Autodesk Inventor part; units mm, degrees
ref_plane "Work Plane1" through (0, 65, -37.4166) normal (0, 0, 1) x (1, 0, 0)
ref_plane "Work Plane2" through (0, 0, -75) normal (0, 0, 1) x (1, 0, 0)
ref_plane "Work Plane3" through (65, 0, -37.4166) normal (1, 0, 0) x (0, 1, 0)
sketch "Sketch1" plane through (0, 0, 0) normal (0, 0, 1) x (1, 0, 0)
  line L0 (65, -65) -> (-65, -65)
  line L1 (-65, -65) -> (-65, 65)
  line L2 (-65, 65) -> (65, 65)
  line L3 (65, 65) -> (65, -65)
  line L4 (65, -65) -> (-65, 65) construction
  line L5 (-65, -65) -> (65, 65) construction
  point P0 (0, 0)
  dimension "d0" = 130
  dimension "d1" = 130
extrude "Extrusion1" add sketch "Sketch1" against normal blind 100
sketch "Sketch2" plane through (0, 0, 0) normal (0, 0, 1) x (1, 0, 0)
  arc A0 (0, 75) -> (0, -75) centre (0, 0) ccw
  line L0 (0, 0) -> (0, 75) construction
  line L1 (0, 0) -> (75, 0) construction
  line L2 (0, 0) -> (0, -75) construction
  line L3 (0, 75) -> (0, -75)
  dimension "d4" = 75
  dimension "d5" = 90
  dimension "d6" = 180
revolve "Revolution1" cut sketch "Sketch2" angle 180 about axis through (0, 75, 0) along (0, -1, 0)
ref_plane "Work Plane1" through (0, 65, -37.4166) normal (0, 0, 1) x (1, 0, 0)
sketch "Sketch3" plane through (0, 65, -37.4166) normal (0, 0, 1) x (1, 0, 0)
  line L0 (-65, -130) -> (65, -130)
  line L1 (65, -130) -> (65, 0)
  line L2 (65, 0) -> (-65, 0)
  line L3 (-65, 0) -> (-65, -130)
  line L4 (-65, -130) -> (65, 0) construction
  line L5 (65, -130) -> (-65, 0) construction
  point P0 (0, -65)
  dimension "d8" = 130
  dimension "d9" = 130
extrude "Extrusion2" cut sketch "Sketch3" along normal blind 100
sketch "Sketch4" plane through (0, 65, -37.4166) normal (0, 0, 1) x (1, 0, 0)
  line L0 (-65, -130) -> (65, -130)
  line L1 (65, -130) -> (65, 0)
  line L2 (65, 0) -> (-65, 0)
  line L3 (-65, 0) -> (-65, -130)
  line L4 (-65, -130) -> (65, 0) construction
  line L5 (65, -130) -> (-65, 0) construction
  line L6 (-70, -135) -> (70, -135)
  line L7 (70, -135) -> (70, 5)
  line L8 (70, 5) -> (-70, 5)
  line L9 (-70, 5) -> (-70, -135)
  arc A0 (65, -65) -> (0, 0) centre (0, -65) ccw
  line L10 (-70, -135) -> (70, 5) construction
  line L11 (70, -135) -> (-70, 5) construction
  dimension "d12" = 130
  dimension "d13" = 130
  dimension "d14" = 140
  dimension "d15" = 140
extrude "Extrusion3" add sketch "Sketch4" against normal blind 50
sketch "Sketch5" plane through (-65, 65, -100) normal (0, 1, 0) x (1, 0, 0)
  line L0 (0, 0) -> (130, 0)
  line L1 (130, 0) -> (130, -12.5834)
  line L2 (130, -12.5834) -> (0, -12.5834)
  line L3 (0, -12.5834) -> (0, 0)
  point P0 (65, -100)
extrude "Extrusion4" cut sketch "Sketch5" against normal blind 130
ref_plane "Work Plane2" through (0, 0, -75) normal (0, 0, 1) x (1, 0, 0)
sketch "Sketch6" plane through (0, 0, -75) normal (0, 0, 1) x (1, 0, 0)
  circle A0 centre (0, 0) radius 30
  dimension "d20" = 60
extrude "Extrusion5" cut sketch "Sketch6" against normal blind 30 and the other way blind 30
sketch "Sketch7" plane through (0, 0, 0) normal (0, 1, 0) x (-1, 0, 0)
  circle A0 centre (0, 0) radius 80
  circle A1 centre (0, 0) radius 150
  dimension "d25" = 160
  dimension "d26" = 300
extrude "Extrusion6" cut sketch "Sketch7" against normal blind 100 and the other way blind 100
sketch "Sketch8" plane through (0, 0, 0) normal (1, 0, 0) x (0, 1, 0)
  point P0 (0, 0)
ref_plane "Work Plane3" through (65, 0, -37.4166) normal (1, 0, 0) x (0, 1, 0)
sketch "Sketch10" plane through (0, 65, -37.4166) normal (0, 0, 1) x (1, 0, 0)
  circle A0 centre (-60.1041, -4.8959) radius 2
  point P0 (0, -65)
  dimension "d36" = 4
  dimension "d37" = 85
  dimension "d38" = 60.1041
sketch "Sketch11" plane through (0, 65, -37.4166) normal (0, 0, 1) x (1, 0, 0)
  circle A0 centre (60.1041, -4.8959) radius 2
  point P0 (0, -65)
  dimension "d39" = 4
  dimension "d40" = 85
  dimension "d41" = 60.1041
sketch "Sketch12" plane through (0, 65, -37.4166) normal (0, 0, 1) x (1, 0, 0)
  circle A0 centre (-60.1041, -125.1041) radius 2
  point P0 (0, -65)
  dimension "d42" = 4
  dimension "d43" = 85
  dimension "d44" = 60.1041
sketch "Sketch13" plane through (0, 65, -37.4166) normal (0, 0, 1) x (1, 0, 0)
  circle A0 centre (60.1041, -125.1041) radius 2
  point P0 (0, -65)
  dimension "d45" = 4
  dimension "d46" = 85
  dimension "d47" = 60.1041
hole "Hole1" at (-60.1041, 60.1041, -37.4166) direction (0, 0, -1) diameter 4 end through all counterbore diameter 12.5 counterbore depth 4
hole "Hole2" at (60.1041, 60.1041, -37.4166) direction (0, 0, -1) diameter 4 end through all counterbore diameter 12.5 counterbore depth 4
hole "Hole3" at (-60.1041, -60.1041, -37.4166) direction (0, 0, -1) diameter 4 end through all counterbore diameter 12.5 counterbore depth 4
hole "Hole4" at (60.1041, -60.1041, -37.4166) direction (0, 0, -1) diameter 4 end through all counterbore diameter 12.5 counterbore depth 4
thread "Thread1"
thread "Thread2"
thread "Thread3"
thread "Thread4"
ref_plane "Work Plane4" through (-70, 30, -37.4166) normal (0, 1, 0) x (1, 0, 0)
ref_plane "Work Plane5" through (0, 0, -65) normal (0, 0, 1) x (1, 0, 0)
sketch "Sketch16" plane through (0, 0, 0) normal (0, 1, 0) x (-1, 0, 0)
  circle A0 centre (0, 0) radius 80
  circle A1 centre (0, 0) radius 150
  dimension "d96" = 160
  dimension "d97" = 300
extrude "Extrusion10" cut sketch "Sketch16" along normal blind 100 and the other way blind 100
ref_plane "Work Plane6" through (-70, -30, -37.4166) normal (0, 1, 0) x (1, 0, 0)
ref_plane "Work Plane7" through (0, 0, -80) normal (0, 0, 1) x (1, 0, 0)
sketch "Sketch22" plane through (0, 0, -80) normal (0, 0, 1) x (1, 0, 0)
  circle A0 centre (0, 0) radius 35
  dimension "d131" = 70
extrude "Extrusion15" cut sketch "Sketch22" along normal blind 7
equation "\"d0\" = d1"
equation "\"d9\" = d8"
properties part number "Custom Mirror Design Part 2"
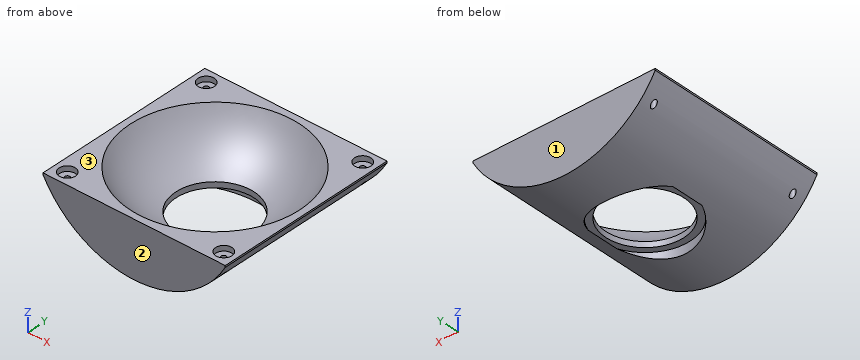
Geometry check sheet. Reference: the model listing, model coordinates, mm. Face numbers are marked on the shaded views. Give positions to 0.01 mm unless a question says otherwise; leave off trailing zeros. Write each loop counter-clockwise with the first axis right and the second up, starting at its lowest first coordinate (ties: lowest second). Pieces come first, ordered by that corner, then holes. Notation, with made-up numbers: (-22.75, 8.25) - (21.25, 8.25) arc R12 cw to (21.25, 18.25) - close; hole circle Ø1 at (-25, 19). An arc over 180 degrees is marked (long way). Put each result on its own line as item: value.
1. Draft check along Y on the marked faces 1, 2 and 3. Enter one of: +Y half, -Y half, draft (parallel to the pull), parting line (faces both ways), or undercut.
Ans:
face 1: +Y half
face 2: -Y half
face 3: draft
2. Sectioned sample at C-C, the plane z = -66.5. Enter the section's corners in (x, y).
Ans:
outline: (-44.47, -70) - (44.47, -70) - (44.47, 70) - (-44.47, 70) - close; hole circle Ø69.36 at (0, 0)
3. Sectioned sample at A-A, the plane y = 0. Enter the section's corners in (x, z), plus the area to 3 significant figures.
Ans:
outline: (-70, -38.73) arc R80 ccw to (-32.73, -73) - (-30, -73) - (-30, -68.74) arc R75 cw to (-65, -37.42) - (-70, -37.42) - close; (30, -73) - (32.73, -73) arc R80 ccw to (70, -38.73) - (70, -37.42) - (65, -37.42) arc R75 cw to (30, -68.74) - close
area: 515 mm²
4. Go/stop test with flat-tipped pins: pin 1 (11 mm diameter, centred on x = 60.1, y = 60.1, fed in from +Z); pin 2 (4 mm diameter, centred on x = 14, y = 28.5, fed in from +Z); pin 3 (8 mm diameter, centred on y = -8, z = -50, fed in from +X). Record where each tip stops, or that it passes through.
Ans:
pin 1: stops at z = -41.42
pin 2: stops at z = -66.98
pin 3: stops at x = 65.45
5. Thickness scan on line 1 (X direction, y = 40.5, z = -53.5); line 2 (Y direction, x = 46, z = -48); line 3 (Y direction, x = 11, z = -64.5). Record the ranges inside material, lowest first.
Ans:
line 1: x = -59.48 to -33.5, 33.5 to 59.48
line 2: y = -70 to -34.71, 34.71 to 70
line 3: y = -70 to -36.66, 36.66 to 70
6. Sectioned sample at D-D, the plane y = 21.5. Enter the section's corners in (x, z).
Ans:
outline: (-70, -38.73) arc R80 ccw to (-27.62, -75.08) - (-27.62, -73) - (-20.92, -73) - (-20.92, -68.74) arc R71.85 cw to (-61.34, -37.42) - (-70, -37.42) - close; (20.92, -73) - (27.62, -73) - (27.62, -75.08) arc R80 ccw to (70, -38.73) - (70, -37.42) - (61.34, -37.42) arc R71.85 cw to (20.92, -68.74) - close
7. Sectioned sample at B-B, the plane x = 0. Enter the section's corners in (y, z), plus the area to 3 significant figures.
Ans:
outline: (-70, -80) - (-35, -80) - (-35, -73) - (-30, -73) - (-30, -68.74) arc R75 cw to (-65, -37.42) - (-70, -37.42) - close; (30, -73) - (35, -73) - (35, -80) - (70, -80) - (70, -37.42) - (65, -37.42) arc R75 cw to (30, -68.74) - close
area: 2,000 mm²
